Verification items for the finished model (mm, model axes). A direction names the side the tool comes from. Round coordinates to 2 decimals unless told otherwise and drop trailing zeros. Order: outer loops, then holes, each group sorted by start corner. A loop starts at its lowest first (then second) coordinate and runs counter-clockwise, first axis right, second up. Notation, with made-up numbers: M 22,26.5 L 51,26.5 A21 cw 51,35.5 Z; hole C -19.75,72.5 d4. An arc over 180 degrees is marked long. Answer as a JSON object with one key per item and string values. Group by question number.
Autodesk Inventor part; units mm, degrees
ref_plane "Arbeitsebene1" through (0, 0, -34) normal (0, 0, 1) x (1, 0, 0)
ref_plane "Arbeitsebene2" through (-22, 0, 0) normal (1, 0, 0) x (0, 1, 0)
ref_plane "XZ Plane" through (0, 0, 0) normal (0, 1, 0) x (-1, 0, 0)
sketch "Skizze1" plane through (0, 0, 0) normal (0, 1, 0) x (-1, 0, 0)
  line L0 (0, 0) -> (44, 0)
  line L1 (44, 0) -> (44, -68)
  line L2 (44, -68) -> (0, -68)
  line L3 (0, -68) -> (0, 0)
  dimension "d0" = 44
  dimension "d1" = 68
extrude "Extrusion1" add sketch "Skizze1" along normal blind 8
sketch "Skizze2" plane through (-44, 0, 0) normal (0, 0, 1) x (1, 0, 0)
  line L0 (44, 0) -> (44, 8)
  point P0 (38, 4)
  point P1 (6, 4)
  point P2 (44, 4)
  dimension "d4" = 32
  dimension "d5" = 6
hole "Bohrung1" at (-6, 4, 0) at (-38, 4, 0) direction (0, 0, -1) diameter 3.242 depth 10
ref_plane "Arbeitsebene1" through (0, 0, -34) normal (0, 0, 1) x (1, 0, 0)
mirror "Spiegeln1" about plane through (0, 0, -34) normal (0, 0, 1) of "Bohrung1"
sketch "Skizze3" plane through (-44, 0, -68) normal (-1, 0, 0) x (0, 0, 1)
  line L0 (68, 0) -> (68, 8)
  point P0 (52, 4)
  point P1 (16, 4)
  point P2 (68, 4)
  dimension "d21" = 16
  dimension "d22" = 36
hole "Bohrung2" at (-44, 4, -16) at (-44, 4, -52) direction (1, 0, 0) diameter 3.242 depth 10
ref_plane "Arbeitsebene2" through (-22, 0, 0) normal (1, 0, 0) x (0, 1, 0)
mirror "Spiegeln2" about plane through (-22, 0, 0) normal (1, 0, 0) of "Bohrung2"
properties part number "1013"
Q1. Tool access check on faces 1 (the face through (-5.07, 3.379, -50.503)), 2 (the face through (-38, 4, -10)), 3 (the face through (-7.582, 4.351, -62.93)), 4 (the face through (-38.93, 4.621, -50.503)). Record the directions out of +Z, -Z, +X, -X, +Y, -Y that give a thin tool (end or side, any length) a straight path to the whole face; none if there is none.
Q2. Cross-section at A-A, the plane x = -6. Record the cut outline in (y, z), then the cut area to 3 significant figures.
Q3. Thickness scan on line 1 (X direction, y = 4, z = -3); line 2 (Z direction, x = -3.25, y = 4); line 3 (Y direction, x = -38, z = -61.25). Record the ranges inside material, lowest first. Write a range as from..to.
Q4. Cross-section at C-C, the plane z = -16. Record the cut outline in (x, y).
Q5. Gauge pin test, flat ends, axial feed: pin 1 Ø1 at (x, y) = (-37.5, 4) entering from -Z; pin 2 Ø1 at (x, y) = (-6, 5) entering from +Z; pin 3 Ø1 at (y, z) = (4.5, -16) entering from +X. Record the tip position at first contact, or that the pin passes through.
Q6. Cross-section at B-B, the plane z = -6. Record the cut outline in (x, y), then the cut area to 3 significant figures.
Q7. Release check for a two-part mould opening along Y. For faces 5 (the face through (-22, 4, 0)), 6 (the face through (-22, 8, -34)), 7 (the face through (-6, 4, -58)) record: released by +Y, released by -Y, zero draft, split by the parting line, or undercut.
Conclusion:
{
 "1": {"face 1": "+X", "face 2": "+Z", "face 3": "-Z", "face 4": "-X"},
 "2": {"outline": "M 0,-68 L 2.38,-68 L 2.38,-58 L 5.62,-58 L 5.62,-68 L 8,-68 L 8,0 L 5.62,0 L 5.62,-10 L 2.38,-10 L 2.38,0 L 0,0 Z; hole C 4,-52 d3.24; hole C 4,-16 d3.24", "area": "463 mm2"},
 "3": {"line 1": "-44..-39.62, -36.38..-7.62, -4.38..0", "line 2": "-68..-53.62, -50.38..-17.62, -14.38..0", "line 3": "0..2.38, 5.62..8"},
 "4": {"outline": "M -44,0 L 0,0 L 0,2.38 L -10,2.38 L -10,5.62 L 0,5.62 L 0,8 L -44,8 L -44,5.62 L -34,5.62 L -34,2.38 L -44,2.38 Z"},
 "5": {"pin 1": "z = -58", "pin 2": "z = -10", "pin 3": "x = -10"},
 "6": {"outline": "M -44,0 L 0,0 L 0,8 L -44,8 Z; hole C -38,4 d3.24; hole C -6,4 d3.24", "area": "335 mm2"},
 "7": {"face 5": "zero draft", "face 6": "released by +Y", "face 7": "undercut"}
}
